Verification items for this drawing (mm, ordinates from the low corner). A direction names the side the tool comes from. Round coordinates to 2 decimals unless told otherwise and drop trailing zeros. Loops run counter-clockwise (first coordinate to the right, second up) from the corner with the lowest first, then second, coordinate; pieces in that order, holes last. Notation, with made-up numbers: (-34.75, -10) -> (-3.75, -10) arc R36 cw to (-3.75, 28) -> close; hole circle Ø5 at (-22, 0.5). An arc over 180 degrees is marked (long way). One line per item, written item: value. Start each with the question number.
1. Set-up check for the marked faces 1 and 2: record each of +Z, -Z, +X, -X, +Y, -Y from which the full face is reachable in a straight line by a thin tool's end or side.
2. Cross-section at D-D on z = 22. Record the cut outline in (x, y).
3. Cross-section at B-B on x = 18. Record the cut outline in (y, z).
4. Material ranges on L1, parallel to Z at x = 4.5, y = 5.25; L2, parallel to Y at x = 13.75, z = 65; L3, parallel to Y at x = 14.25, z = 65, recorded low to high.
5. Go/stop test with flat-tipped pins: pin 1 (1 mm diameter, centred on y = 13.5, z = 50.5, fed in from +X); pin 2 (1 mm diameter, centred on y = 12, z = 40.5, fed in from +X); pin 3 (6 mm diameter, centred on x = 12.5, z = 36.5, fed in from -Y). Record where each tip stops, or that it passes through.
6. Cross-section at A-A on y = 10. Record the cut outline in (x, z), then the cut area to 3 significant figures.
7. Cross-section at C-C on y = 7. Record the cut outline in (x, z), then the cut area to 3 significant figures.
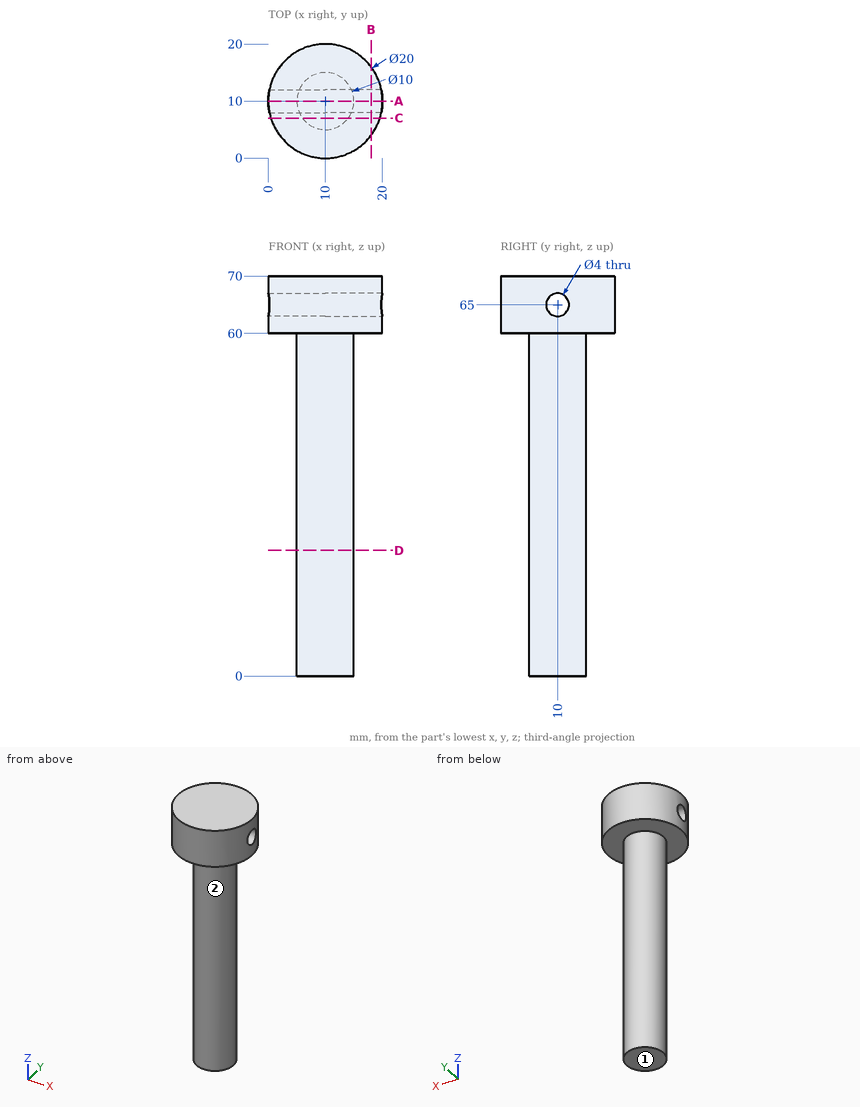
Taken from the geometry:
1. face 1: -Z, +X, -X, +Y, -Y
1. face 2: -Z
2. outline: circle Ø10 at (10, 10)
3. outline: (4, 60) -> (16, 60) -> (16, 70) -> (4, 70) -> close; hole circle Ø4 at (10, 65)
4. L1: z = 60 to 70
4. L2: y = 0.73 to 8, 12 to 19.27
4. L3: y = 0.95 to 8, 12 to 19.05
5. pin 1: stops at x = 14
5. pin 2: stops at x = 14.77
5. pin 3: stops at y = 5
6. outline: (0, 60) -> (5, 60) -> (5, 0) -> (15, 0) -> (15, 60) -> (20, 60) -> (20, 63) -> (0, 63) -> close; (0, 67) -> (20, 67) -> (20, 70) -> (0, 70) -> close
6. area: 720 mm2
7. outline: (0.46, 60) -> (6, 60) -> (6, 0) -> (14, 0) -> (14, 60) -> (19.54, 60) -> (19.54, 70) -> (0.46, 70) -> close
7. area: 671 mm2
